The model under review builds one solid part; all positions refer to its coordinate system, in mm. A direction names the side the tool comes from. Coordinates: 2 decimals unless noted, no trailing zeros. Loops run counter-clockwise (first coordinate to the right, second up) from the corner with the lowest first, then second, coordinate; pieces in that order, holes last. Notation, with made-up numbers: M -9.5,76 L 35.5,76 A16 cw 35.5,105 Z; hole C -22.5,17 d11. An arc over 180 degrees is marked long. Use one line per item in the form item = value.
```python
from build123d import *

# Parameters (mm, degrees)
F2_DEPTH = 25.4
F3_W     = 13.6997364461
F3_H     = 10.9366187826
F4_DEPTH = 25.4
F7_DEPTH = 50.8


with BuildPart() as f2:
    # F0 (on Front) → F2 (new body)
    with BuildSketch(Plane.XZ):
        Polygon((-43.6756652357, 82.9696333554), (-43.6756652357, -69.4303666446), (7.1243347643, -44.0303666446), (7.1243347643, 82.9696333554), align=None)
    extrude(amount=F2_DEPTH)

    # F3 (on face) → F4 (join)
    with BuildSketch(Plane.YZ.offset(7.1243347643)):
        Polygon((-8.0585619435, 0), (-8.9219789952, 10.9366187826), (-11.7082890579, 10.9366187826), (-16.8076753616, 0), align=None)
        Polygon((-16.8076753616, 0), (-11.7082890579, 10.9366187826), (-16.8076753616, 10.9366187826), align=None)
        Polygon((-16.8076753616, 10.9366187826), (-11.7082890579, 10.9366187826), (0, 36.0473059118), (-16.8076753616, 41.0203114152), align=None)
        with Locations((-23.6575435847, 5.4683093913)):
            Rectangle(F3_W, F3_H)
    extrude(amount=F4_DEPTH)

    # F6 (on face) → F7 (cut)
    with BuildSketch(Plane.XZ.offset(25.4)):
        Polygon((4.574265326, 8.322226192), (-39.875734674, 8.322226192), (-41.4155621324, -38.6425375293), (4.574265326, -38.6425375293), align=None)
    extrude(amount=-F7_DEPTH, mode=Mode.SUBTRACT)


solid = f2.part
```
1. The part is to be moulded in two halves that separate along Z. For faces 1 (the face through (20, -16.808, 26)), 2 (the face through (20, -19, 0)), 3 (the face through (19.647, -8.484, 5.392)), say which applies: pulls with the +Z half, pulls with the -Z half, needs draft (parallel to the pull), parting line crosses it, or undercut.
Response values:
face_1 = needs draft
face_2 = pulls with the -Z half
face_3 = undercut
2. Add section D-D (z = -5). State the section outline as (x, y) points, then the cut area to 3 significant figures.
Response values:
outline = M -43.68,-25.4 L -40.31,-25.4 L -40.31,0 L -43.68,0 Z; M 4.57,-25.4 L 7.12,-25.4 L 7.12,0 L 4.57,0 Z
area = 150 mm^2
3. Add section C-C (x = 3). State the section outline as (y, z) points, then the cut area to 3 significant figures.
Response values:
outline = M -25.4,-46.09 L 0,-46.09 L 0,-38.64 L -25.4,-38.64 Z; M -25.4,8.32 L 0,8.32 L 0,82.97 L -25.4,82.97 Z
area = 2,090 mm^2
4. Machinability: for faces 4 (the face through (7.124, -28, 6)), 5 (the face through (19.647, -5.936, 23.316)), 6 (the face through (4.574, -13, -15)), which of the approach directions +Z, -Z, +X, -X, +Y, -Y give a long, thin tool a straight path to every point of the face, cutting with its end or side? Answer none if there is none.
Response values:
face_4 = +Z, -Z, -X, -Y
face_5 = +X, +Y
face_6 = +Y, -Y
5. Add section B-B (y = -24). State the section outline as (x, z) points, then the cut area to 3 significant figures.
Response values:
outline = M -43.68,-69.43 L 7.12,-44.03 L 7.12,0 L 32.52,0 L 32.52,10.94 L 7.12,10.94 L 7.12,82.97 L -43.68,82.97 Z; hole M -41.42,-38.64 L 4.57,-38.64 L 4.57,8.32 L -39.88,8.32 Z
area = 5,250 mm^2
6. Wall thickness on line 1 along X through (y, z) = (-10, -56); line 2 along Y through (x, z) = (-40, 55); line 3 along Z through (x, y) = (-36.5, -21): over which ranges is each line inside the solid? List them lowest first. Write a range as from..to.
Response values:
line_1 = -43.68..-16.81
line_2 = -25.4..0
line_3 = -65.84..-38.64, 8.32..82.97
7. Insertion check: P1, Ø5, axis at x = 21.5, z = 28, coming from the -Y side; P2, Ø5, axis at y = -15.5, z = -25, coming from the +X side; P3, Ø2, axis at x = 24.5, y = -10.5, coming from the +Z side. Each pin has a flat end and moves straight along its axis. Give the tip position at first contact, or say it passes through.
Response values:
P1 = -16.81
P2 = 7.12
P3 = 39.45
8. Add section A-A (x = 22.5). State the section outline as (y, z) points, then the cut area to 3 significant figures.
Response values:
outline = M -30.51,0 L -8.06,0 L -8.92,10.94 L -11.71,10.94 L 0,36.05 L -16.81,41.02 L -16.81,10.94 L -30.51,10.94 Z
area = 558 mm^2
